from build123d import *

# Parameters (mm, degrees)
SKETCH1_W           = 16
SKETCH1_H           = 16
SKETCH1_W_2         = 12.8
SKETCH1_H_2         = 12.8
BOSS_EXTRUDE1_DEPTH = 8
SKETCH2_W           = 16
SKETCH2_H           = 16
BOSS_EXTRUDE2_DEPTH = 1.6
SKETCH3_R           = 2.4
BOSS_EXTRUDE3_DEPTH = 1.6
SKETCH4_R           = 3.25
CUT_EXTRUDE1_DEPTH  = 1.6
SKETCH7_W           = 3
SKETCH7_H           = 6
CUT_EXTRUDE2_DEPTH  = 1.6


with BuildPart() as part:
    # Sketch1 → Boss-Extrude1 (new body)
    with BuildSketch(Plane(origin=(0, 0, 0), x_dir=(1, 0, 0), z_dir=(0, 1, 0))):
        with Locations((8, 8)):
            Rectangle(SKETCH1_W, SKETCH1_H)
        with Locations((8, 8)):
            Rectangle(SKETCH1_W_2, SKETCH1_H_2, mode=Mode.SUBTRACT)
    extrude(amount=BOSS_EXTRUDE1_DEPTH)

    # Sketch2 → Boss-Extrude2 (add)
    with BuildSketch(Plane(origin=(0, 8, 0), x_dir=(1, 0, 0), z_dir=(0, 1, 0))):
        with Locations((8, 8)):
            Rectangle(SKETCH2_W, SKETCH2_H)
    extrude(amount=BOSS_EXTRUDE2_DEPTH)

    # Sketch3 → Boss-Extrude3 (add)
    with BuildSketch(Plane(origin=(0, 9.6, 0), x_dir=(1, 0, 0), z_dir=(0, 1, 0))):
        with Locations((12, 4)):
            Circle(SKETCH3_R)
        with Locations((4, 4)):
            Circle(SKETCH3_R)
        with Locations((4, 12)):
            Circle(SKETCH3_R)
        with Locations((12, 12)):
            Circle(SKETCH3_R)
    extrude(amount=BOSS_EXTRUDE3_DEPTH)

    # Sketch4 → Cut-Extrude1 (cut)
    with BuildSketch(Plane.ZY):
        with Locations((-8, 4.8)):
            Circle(SKETCH4_R)
    extrude(amount=-CUT_EXTRUDE1_DEPTH, mode=Mode.SUBTRACT)

    # Sketch7 → Cut-Extrude2 (cut)
    with BuildSketch(Plane(origin=(16, 0, 0), x_dir=(0, 0, -1), z_dir=(1, 0, 0))):
        with Locations((8, 4.8)):
            Rectangle(SKETCH7_W, SKETCH7_H)
    extrude(amount=-CUT_EXTRUDE2_DEPTH, mode=Mode.SUBTRACT)


solid = part.part
For this review, take the finished solid that the model builds, in its own axes (mm). A direction names the side the tool comes from. Round coordinates to 2 decimals unless told otherwise and drop trailing zeros. Loops run counter-clockwise (first coordinate to the right, second up) from the corner with the lowest first, then second, coordinate; pieces in that order, holes last. Notation, with made-up numbers: (56.25, 31.5) - (81.25, 31.5) arc R34 cw to (81.25, 68.5) - close; hole circle Ø1 at (-23, 41.25). An arc over 180 degrees is marked (long way). One line per item, written item: value. Start each with the question number.
Item 1: Take a section at C-C (x = 4). Give the boundary of the cut face in (y, z).
Item 2: Take a section at D-D (z = -10.5). Give the boundary of the cut face in (x, y), plus the area to 3 significant figures.
Item 3: Take a section at B-B (y = 4.8). Give the boundary of the cut face in (x, z).
Item 4: For L1, parallel to Y at x = 0.55, z = -8; L2, parallel to X at y = 0.75, z = -3.5; L3, parallel to Z at x = 15.25, y = 3.75, list the stretches that pass through material, from the lowest coordinate up.
Item 5: Clearance check with flat-ended pins moving along their axes: pin 1 Ø6.5 at (x, z) = (11, -9) entering from -Y; pin 2 Ø3 at (x, z) = (9.5, -8) entering from +Y. State where each tip first meets the part, or that it passes through.
Item 6: For faces 4 (the cylindrical face through (0.789, 4.943, -11.247)), 5 (the cylindrical face through (13.29, 10.389, -6.024)), 6 (the flat face through (15, 7.8, -8)), list the 3-axis set-ups (+Z, -Z, +X, -X, +Y, -Y) from which the entire face can be reached by the end or side of a thin tool; tool diameter is ignored.
Item 7: The part is to be moulded in two halves that separate along X. For faces 1 (the flat face through (16, 5, -10)), 2 (the flat face through (1.6, 1, -8)), 3 (the flat face through (12, 11.2, -4)), say which applies: +X half, -X half, draft (parallel to the pull), parting line (faces both ways), or undercut.
Item 8: Take a section at A-A (z = -8). Give the boundary of the cut face in (x, y).
Answer below:
1. outline: (0, -16) - (9.6, -16) - (9.6, -14.4) - (11.2, -14.4) - (11.2, -9.6) - (9.6, -9.6) - (9.6, -6.4) - (11.2, -6.4) - (11.2, -1.6) - (9.6, -1.6) - (9.6, 0) - (0, 0) - (0, -1.6) - (8, -1.6) - (8, -14.4) - (0, -14.4) - close
2. outline: (0, 0) - (1.6, 0) - (1.6, 2.72) - (0, 2.72) - close; (0, 6.88) - (1.6, 6.88) - (1.6, 8) - (14.4, 8) - (14.4, 0) - (16, 0) - (16, 9.6) - (13.87, 9.6) - (13.87, 11.2) - (10.13, 11.2) - (10.13, 9.6) - (5.87, 9.6) - (5.87, 11.2) - (2.13, 11.2) - (2.13, 9.6) - (0, 9.6) - close
2. area: 56.5 mm2
3. outline: (0, -16) - (16, -16) - (16, -9.5) - (14.4, -9.5) - (14.4, -14.4) - (1.6, -14.4) - (1.6, -11.25) - (0, -11.25) - close; (0, -4.75) - (1.6, -4.75) - (1.6, -1.6) - (14.4, -1.6) - (14.4, -6.5) - (16, -6.5) - (16, 0) - (0, 0) - close
4. L1: y = 0 to 1.55, 8.05 to 9.6
4. L2: x = 0 to 1.6, 14.4 to 16
4. L3: z = -16 to -9.5, -6.5 to 0
5. pin 1: stops at y = 8
5. pin 2: stops at y = 9.6
6. face 4: -X
6. face 5: +Y
6. face 6: +X
7. face 1: +X half
7. face 2: undercut
7. face 3: draft
8. outline: (0, 0) - (1.6, 0) - (1.6, 1.55) - (0, 1.55) - close; (0, 8.05) - (1.6, 8.05) - (1.6, 8) - (14.4, 8) - (14.4, 7.8) - (16, 7.8) - (16, 9.6) - (0, 9.6) - close; (14.4, 0) - (16, 0) - (16, 1.8) - (14.4, 1.8) - close
